```python
from build123d import *

# Parameters (mm, degrees)
MAINPROFILES_W         = 0.4
MAINPROFILES_H         = 4
CONNECTIONACCESS_REACH = 11.742
CONNECTIONACCESSS_W    = 3
CONNECTIONACCESSS_H    = 4.6
ENDPROFILES_W          = 4
ENDPROFILES_H          = 0.4
ENDCONNECTIONS_W       = 2
ENDCONNECTIONS_H       = 0.4
LOCKINGTABS_W          = 1.6
LOCKINGTABS_H          = 0.4
LTCUT_REACH            = 10.24
LTCUTF_R               = 0.2
MPC_SIZE               = 0.8


with BuildPart() as part:
    # MainProfile: sweep along a path in MainProfilePath
    with BuildLine(Plane.XY) as mainprofile_path:
        Line((0, 0), (-1, 2.291287847))
        ThreePointArc((-1, 2.291287847), (-1.081718762, 2.513588866), (-1.136585228, 2.743991492))
        Line((-1.136585228, 2.743991492), (-1.570705672, 5.206010875))
        ThreePointArc((-1.570705672, 5.206010875), (-1.395695024, 5.859159505), (-0.78285947, 6.144929417))
        Line((-0.78285947, 6.144929417), (5.21714053, 6.144929417))
        ThreePointArc((5.21714053, 6.144929417), (6.902596795, 4.22303489), (4.777148154, 2.802855512))
        Line((4.777148154, 2.802855512), (1.879370675, 3.579312647))
        ThreePointArc((1.879370675, 3.579312647), (1.749961152, 3.596349734), (1.62055163, 3.579312647))
    # MainProfileS → MainProfile (sweep)
    with BuildSketch(Plane(origin=(0, 0, 0), x_dir=(0.9165151389911679, 0.4000000000000004, 0), z_dir=(-0.4000000000000004, 0.9165151389911679, 0))):
        Rectangle(MAINPROFILES_W, MAINPROFILES_H)
    sweep(path=mainprofile_path.line)

    # ConnectionAccessS → ConnectionAccess (cut, up to next)
    with BuildSketch(Plane(origin=(0, 0, 0), x_dir=(0, 0, -1), z_dir=(1, 0, 0)), mode=Mode.PRIVATE) as connectionaccess_sk1:
        with Locations((0, 4.044929417)):
            Rectangle(CONNECTIONACCESSS_W, CONNECTIONACCESSS_H)
    connectionaccess_tool1 = extrude(connectionaccess_sk1.sketch, amount=-CONNECTIONACCESS_REACH, mode=Mode.PRIVATE) & part.part
    add(connectionaccess_tool1.solids().sort_by_distance((0, 4.044929, 0))[0], mode=Mode.SUBTRACT)

    # EndProfile: sweep along a path in EndProfilePath
    with BuildLine(Plane.XY) as endprofile_path:
        Line((1.62055163, 3.579312647), (-0.311300023, 3.061674557))
    # EndProfileS → EndProfile (sweep)
    with BuildSketch(Plane(origin=(2.406823416, 0.644906391, 0), x_dir=(0, 0, 1), z_dir=(-0.9659258262890702, -0.2588190451025136, 0))):
        with Locations((0, 3.037920901)):
            Rectangle(ENDPROFILES_W, ENDPROFILES_H)
    sweep(path=endprofile_path.line)

    # EndConnection: sweep along a path in EndConnectionPath
    with BuildLine(Plane.XY) as endconnection_path:
        Line((-0.311300023, 3.061674557), (-1.277225849, 2.802855512))
    # EndConnectionS → EndConnection (sweep)
    with BuildSketch(Plane(origin=(0.474971764, 0.127268301, 0), x_dir=(0, 0, 1), z_dir=(-0.9659258262890702, -0.2588190451025135, 0))):
        with Locations((0, 3.037920901)):
            Rectangle(ENDCONNECTIONS_W, ENDCONNECTIONS_H)
    sweep(path=endconnection_path.line)

    # LockingTab: sweep along a path in LockingTabPath
    with BuildLine(Plane.XY) as lockingtab_path:
        Line((-1.398843786, 5.368246688), (-0.1, 6.118134498))
        ThreePointArc((-0.1, 6.118134498), (-0.051763809, 6.138114582), (0, 6.144929417))
    # LockingTabS → LockingTab (sweep)
    with BuildSketch(Plane.ZY):
        with Locations((0, 6.144929417)):
            Rectangle(LOCKINGTABS_W, LOCKINGTABS_H)
    sweep(path=lockingtab_path.line)

    # LTCutS → LTCut (cut, up to next)
    with BuildSketch(Plane(origin=(2.972464708, 6.344929417, 0), x_dir=(-1, 0, 0), z_dir=(0, -1, 0)), mode=Mode.PRIVATE) as ltcut_sk1:
        Polygon((2.972464708, 0.8), (4.471308495, 0.4), (4.471308495, 0.8), align=None)
    ltcut_tool1 = extrude(ltcut_sk1.sketch, amount=LTCUT_REACH, mode=Mode.PRIVATE) & part.part
    ltcut = ltcut_tool1.solids().sort_by_distance((-0.999229, 6.344929, -0.666667))[0]
    add(ltcut, mode=Mode.SUBTRACT)

    # LTCutHM: LTCut across plane
    add(ltcut.mirror(Plane.XY), mode=Mode.SUBTRACT)

    # LTCutF
    # the kernel refuses this fillet: 0.2 mm, written as the material it adds along each edge
    with BuildSketch(Plane(origin=(0, 5.560866603, 0.8), x_dir=(0, 0, 1), z_dir=(0, 1, 0))) as ltcutf_piece_1_section:
        with BuildLine():
            CenterArc((LTCUTF_R * 0.768125627693, -LTCUTF_R), LTCUTF_R, 90, 75.05757969)
            Line((-LTCUTF_R * 0.198059812329, -LTCUTF_R * 0.742151797585), (0, 0))
            Line((0, 0), (LTCUTF_R * 0.768125627693, 0))
        make_face()
    ltcutf_piece_1 = extrude(amount=1.168125628, mode=Mode.PRIVATE)
    ltcutf_piece_1 = split(ltcutf_piece_1, bisect_by=Plane(origin=(-0.048441187, 5.916961885, 0.804118212), z_dir=(-0.4999999999999946, 0.8660254037844418, 0)), keep=Keep.TOP, mode=Mode.PRIVATE)
    ltcutf_piece_1 = ltcutf_piece_1 & Plane(origin=(0, 5.944929417, 0.804118212), x_dir=(-0.5000000000000254, 0.8660254037844239, 0), z_dir=(0, 0, -1)) * Cylinder(0.4, 3, mode=Mode.PRIVATE)
    add(ltcutf_piece_1)
    with BuildSketch(Plane(origin=(0, 6.728992231, -0.8), x_dir=(0, 0, -1), z_dir=(0, -1, 0))) as ltcutf_piece_2_section:
        with BuildLine():
            CenterArc((LTCUTF_R * 0.768125627693, -LTCUTF_R), LTCUTF_R, 90, 75.05757969)
            Line((-LTCUTF_R * 0.198059812329, -LTCUTF_R * 0.742151797585), (0, 0))
            Line((0, 0), (LTCUTF_R * 0.768125627693, 0))
        make_face()
    ltcutf_piece_2 = extrude(amount=1.168125628, mode=Mode.PRIVATE)
    ltcutf_piece_2 = split(ltcutf_piece_2, bisect_by=Plane(origin=(0.062272653, 5.98088255, -0.82477541), z_dir=(-0.4999999999999946, 0.8660254037844418, 0)), keep=Keep.TOP, mode=Mode.PRIVATE)
    ltcutf_piece_2 = ltcutf_piece_2 & Plane(origin=(0, 5.944929417, -0.82477541), x_dir=(-0.5000000000000254, 0.8660254037844239, 0), z_dir=(0, 0, -1)) * Cylinder(0.4, 3, mode=Mode.PRIVATE)
    add(ltcutf_piece_2)
    # the kernel refuses this fillet: 0.2 mm, written as the material it takes off along each edge
    with BuildSketch(Plane(origin=(-1.101389565, 4.853040863, 0.506069552), x_dir=(0.8293899797947963, 0.5129525340785382, 0.22134127314713234), z_dir=(-0.49560726984934556, 0.8584169719794723, -0.13226388883618956)), Plane(origin=(-1.101389565, 4.853040863, -0.506069552), x_dir=(0.06613194441810266, -0.11454388773545661, 0.9912145396986104), z_dir=(-0.49560726984934556, 0.8584169719794723, 0.13226388883618956))) as ltcutf_2_piece_1:
        with BuildLine():
            CenterArc((LTCUTF_R * 0.796817292686, LTCUTF_R), LTCUTF_R, 192.903114006, 77.096885994)
            Line((-LTCUTF_R * 0.1779317665, LTCUTF_R * 0.776696906389), (0, 0))
            Line((0, 0), (LTCUTF_R * 0.796817292686, 0))
        make_face()
    extrude(amount=1.200362624, mode=Mode.SUBTRACT)

    # MPC
    mpc_edges = [part.edges().sort_by_distance(p)[0] for p in [
        (0, 0, -2),
        (0, 0, 2),
    ]]
    chamfer(mpc_edges, length=MPC_SIZE)


solid = part.part
```
Part model, mm, in its own coordinate system. A direction names the side the tool comes from. Coordinates: 2 decimals unless noted, no trailing zeros. Loops run counter-clockwise (first coordinate to the right, second up) from the corner with the lowest first, then second, coordinate; pieces in that order, holes last. Notation, with made-up numbers: (-8, 30) - (-1, 30) arc R24 cw to (-1, 48) - close; hole circle Ø8 at (72, -20). An arc over 180 degrees is marked (long way). Write item = value, one per line. Start each with the question number.
Item 1: 3-axis set-ups, long thin cutter, end or side, ignore diameter. For faces 4 (the flat face through (2, 6.345, 0)), 5 (the flat face through (-0.84, 5.92, 0.01)), 6 (the flat face through (-0.213, 0.987, 0.028)), 7 (the flat face through (3.36, 3.39, 0.03)): which of +Z, -Z, +X, -X, +Y, -Y reach the whole face in a straight line?
Item 2: Wall check: L1, parallel to Y at x = 1.75, z = 0.7; L2, parallel to Y at x = 5.25, z = -0.2; L3, parallel to Y at x = 6.75, z = -0.7. Give the ranges that are in metal, low to high. Write a range as from..to.
Item 3: Mould opens along X. For faces 1 (the flat face through (3.256, 3.003, -0.028)), 2 (the cylindrical face through (-1.557, 5.978, -1.746)), 3 (the flat face through (-1.35, 4.2, 1.5)) say: released by +X, released by -X, zero draft, split by the parting line, or undercut.
Item 4: Cut at D-D, the plane z = -1.35. Give the cut face in (x, y).
Item 5: Cut at A-A, the plane z = -0.1. Give the cut face in (x, y).
Item 6: Flat gauge pin, fed straight in: pin 1 Ø1.2 at (x, z) = (3.5, -0.5) entering from -Y. Where does the tip first touch, or does it go through?
Item 7: Cut at B-B, the plane y = 4.75. Give the cut face in (x, z).
Item 8: Cut at C-C, the plane x = 1. Give the cut face in (y, z).
The answers:
q1.face_4 = +Z, -Z, +X, -X, +Y
q1.face_5 = -X, +Y
q1.face_6 = +Z, -Z, +X
q1.face_7 = +Z, -Z
q2.L1 = 3.4..3.8, 5.94..6.34
q2.L2 = 2.55..2.95, 5.94..6.34
q2.L3 = 3.32..5.57
q3.face_1 = undercut
q3.face_2 = released by -X
q3.face_3 = zero draft
q4.outline = (-0.98, 1.74) - (-0.24, 0.06) - (0.12, 0.22) - (-0.54, 1.74) - close; (-0.36, 3.25) - (-0.26, 2.87) - (1.67, 3.39) arc R0.3 cw to (1.83, 3.39) - (4.73, 2.61) arc R1.9 ccw (long way) to (5.22, 6.34) - (0, 6.34) - (0, 5.94) - (5.22, 5.94) arc R1.5 cw (long way) to (4.83, 3) - (1.93, 3.77) arc R0.7 ccw to (1.57, 3.77) - close
q5.outline = (-1.5, 5.54) - (-1.3, 5.2) - (0, 5.94) - (5.22, 5.94) arc R1.5 cw (long way) to (4.83, 3) - (1.93, 3.77) arc R0.7 ccw to (1.57, 3.77) - (-1.33, 3) - (-1.23, 2.61) - (1.67, 3.39) arc R0.3 cw to (1.83, 3.39) - (4.73, 2.61) arc R1.9 ccw (long way) to (5.22, 6.34) - (0, 6.34) arc R0.4 ccw to (-0.2, 6.29) - close; (-0.98, 1.74) - (-0.18, -0.08) - (0.18, 0.08) - (-0.54, 1.74) - close
q6.pin_1 = 2.78
q7.outline = (-1.69, -2) - (-1.29, -2) - (-1.29, -1.5) - (-1.69, -1.5) - close; (-1.69, 1.5) - (-1.29, 1.5) - (-1.29, 2) - (-1.69, 2) - close; (6.69, -2) - (7.09, -2) - (7.09, 2) - (6.69, 2) - close
q8.outline = (3.21, -2) - (3.62, -2) - (3.62, 2) - (3.21, 2) - close; (5.94, -2) - (6.34, -2) - (6.34, 2) - (5.94, 2) - close
